```python
from build123d import *

# Parameters (mm, degrees)
SKETCH004_W                 = 51
SKETCH004_H                 = 35.4
PAD002_DEPTH                = 23.5
THICKNESS001_T              = 2
POCKET002_DEPTH             = 55.001
POCKET003_DEPTH             = 2
POCKET004_DEPTH             = 2
POCKET005_DEPTH             = 2
SKETCH009_W                 = 6
SKETCH009_H                 = 2.4
PAD003_DEPTH                = 0.5
SKETCH010_R                 = 1.2
POCKET006_DEPTH             = 2
SKETCH011_W                 = 10
SKETCH011_H                 = 3
PAD004_DEPTH                = 23.5
SKETCH011_POLARPATTERN_2_W  = 10
SKETCH011_POLARPATTERN_2_H  = 3
PAD004_POLARPATTERN_2_DEPTH = 23.5
SKETCH022_W                 = 10
SKETCH022_H                 = 0.15
POCKET013_DEPTH             = 7.1
SKETCH013_R                 = 1.1
SKETCH013_W                 = 10
SKETCH013_H                 = 3.02
PAD005_DEPTH                = 5
SKETCH014_W                 = 2.2
SKETCH014_H                 = 17.18
SKETCH014_H_2               = 17.78
PAD006_DEPTH                = 2.4
SKETCH019_R                 = 0.6
POCKET010_DEPTH             = 42.301
FILLET001_R                 = 1.85
FILLET002_R                 = 1.5


with BuildPart() as part:
    # Sketch004 → Pad002 (new body)
    with BuildSketch(Plane.XY):
        Rectangle(SKETCH004_W, SKETCH004_H)
    extrude(amount=PAD002_DEPTH)

    # Thickness001
    thickness001_openings = [part.faces().sort_by_distance(p)[0] for p in [
        (0, 0, 0),
    ]]
    offset(amount=THICKNESS001_T, openings=thickness001_openings)

    # Sketch005 (on DatumPlane) → Pocket002 (cut, through all)
    with BuildSketch(Plane.YZ.offset(27.5)):
        with BuildLine():
            Line((17.046003, 7.1), (13.527395, 1.798614))
            ThreePointArc((10.361297, 0.1), (12.157784, 0.551473), (13.527395, 1.798614))
            Line((10.361297, 0.1), (-10.361297, 0.1))
            ThreePointArc((-13.527395, 1.798614), (-12.157784, 0.551473), (-10.361297, 0.1))
            Line((-13.527395, 1.798614), (-17.046003, 7.1))
            Line((-17.046003, 7.1), (-40, 7.1))
            Line((-40, 7.1), (-40, -32.9))
            Line((-40, -32.9), (40, -32.9))
            Line((40, -32.9), (40, 7.1))
            Line((40, 7.1), (17.046003, 7.1))
        make_face()
    extrude(amount=-POCKET002_DEPTH, mode=Mode.SUBTRACT)

    # Sketch006 (on DatumPlane) → Pocket003 (cut)
    with BuildSketch(Plane.YZ.offset(-27.5)):
        with BuildLine():
            ThreePointArc((6.4, 6.5), (6.107107, 7.207107), (5.4, 7.5))
            Line((-5.4, 7.5), (5.4, 7.5))
            ThreePointArc((-5.4, 7.5), (-6.107107, 7.207107), (-6.4, 6.5))
            Line((-6.4, 3.5), (-6.4, 6.5))
            ThreePointArc((-6.4, 3.5), (-6.107107, 2.792893), (-5.4, 2.5))
            Line((5.4, 2.5), (-5.4, 2.5))
            ThreePointArc((5.4, 2.5), (6.107107, 2.792893), (6.4, 3.5))
            Line((6.4, 6.5), (6.4, 3.5))
        make_face()
    extrude(amount=POCKET003_DEPTH, mode=Mode.SUBTRACT)

    # Sketch007 (on DatumPlane) → Pocket004 (cut)
    with BuildSketch(Plane.YZ.offset(27.5)):
        with BuildLine():
            ThreePointArc((-7, 21), (-7.707107, 20.707107), (-8, 20))
            Line((-8, 10), (-8, 20))
            ThreePointArc((-8, 10), (-7.707107, 9.292893), (-7, 9))
            Line((7, 9), (-7, 9))
            ThreePointArc((7, 9), (7.707107, 9.292893), (8, 10))
            Line((8, 20), (8, 10))
            ThreePointArc((8, 20), (7.707107, 20.707107), (7, 21))
            Line((-7, 21), (7, 21))
        make_face()
    extrude(amount=-POCKET004_DEPTH, mode=Mode.SUBTRACT)

    # Sketch008 (on DatumPlane) → Pocket005 (cut)
    with BuildSketch(Plane.XY.offset(25.5)):
        Polygon((-5.5, 15.8), (-4.5, 15.8), (-4.5, 1.8), (4.5, 1.8), (4.5, 15.8), (5.5, 15.8), (5.5, 0.8), (-5.5, 0.8), align=None)
        Polygon((-5.5, -0.8), (5.5, -0.8), (5.5, -15.8), (4.5, -15.8), (4.5, -1.8), (-4.5, -1.8), (-4.5, -15.8), (-5.5, -15.8), align=None)
    extrude(amount=-POCKET005_DEPTH, mode=Mode.SUBTRACT)

    # Sketch009 (on Face4 of Pocket005) → Pad003 (join)
    with BuildSketch(Plane(origin=(0, 0, 23.5), x_dir=(1, 0, 0), z_dir=(0, 0, -1))):
        with Locations((0, -3)):
            Rectangle(SKETCH009_W, SKETCH009_H)
        with Locations((0, 3)):
            Rectangle(SKETCH009_W, SKETCH009_H)
    extrude(amount=PAD003_DEPTH)

    # Sketch010 (on DatumPlane) → Pocket006 (cut)
    with BuildSketch(Plane.XY.offset(25.5)):
        with Locations((19, 3)):
            Circle(SKETCH010_R)
        with Locations((9, 3)):
            Circle(SKETCH010_R)
        with Locations((-9, 3)):
            Circle(SKETCH010_R)
        with Locations((-19, 3)):
            Circle(SKETCH010_R)
        with Locations((-19, -3)):
            Circle(SKETCH010_R)
        with Locations((-9, -3)):
            Circle(SKETCH010_R)
        with Locations((9, -3)):
            Circle(SKETCH010_R)
        with Locations((19, -3)):
            Circle(SKETCH010_R)
    extrude(amount=-POCKET006_DEPTH, mode=Mode.SUBTRACT)

    # Sketch011 (on DatumPlane) → Pad004 (join)
    with BuildSketch(Plane.XY.offset(23.5)):
        with Locations((19.5, -16.2)):
            Rectangle(SKETCH011_W, SKETCH011_H)
    pad004 = extrude(amount=-PAD004_DEPTH)

    # Sketch011 PolarPattern 2 → Pad004 PolarPattern 2 (add)
    with BuildSketch(Plane(origin=(0, 0, 23.5), x_dir=(-1, 0, 0), z_dir=(0, 0, 1))):
        with Locations((19.5, -16.2)):
            Rectangle(SKETCH011_POLARPATTERN_2_W, SKETCH011_POLARPATTERN_2_H)
    pad004_polarpattern_2 = extrude(amount=-PAD004_POLARPATTERN_2_DEPTH)

    # Mirrored: Pad004, Pad004 PolarPattern 2 across Sketch011 V_Axis
    add(pad004.mirror(Plane(origin=(0, 0, 23.5), x_dir=(0, 0, 1), z_dir=(1, 0, 0))))
    add(pad004_polarpattern_2.mirror(Plane(origin=(0, 0, 23.5), x_dir=(0, 0, 1), z_dir=(1, 0, 0))))

    # Sketch022 (on DatumPlane) → Pocket013 (cut)
    with BuildSketch(Plane(origin=(0, 0, 0), x_dir=(-1, 0, 0), z_dir=(0, 0, -1))):
        with Locations((19.5, -17.625)):
            Rectangle(SKETCH022_W, SKETCH022_H)
        with Locations((-19.5, -17.625)):
            Rectangle(SKETCH022_W, SKETCH022_H)
        with Locations((19.5, 17.625)):
            Rectangle(SKETCH022_W, SKETCH022_H)
        with Locations((-19.5, 17.625)):
            Rectangle(SKETCH022_W, SKETCH022_H)
    extrude(amount=-POCKET013_DEPTH, mode=Mode.SUBTRACT)

    # Sketch013 (on DatumPlane) → Pad005 (join)
    with BuildSketch(Plane.XY.offset(23.5)):
        with Locations((-22.86, -8.59)):
            Circle(SKETCH013_R)
        with Locations((22.86, -8.89)):
            Circle(SKETCH013_R)
        with Locations((22.86, 8.89)):
            Circle(SKETCH013_R)
        with Locations((-22.86, 8.59)):
            Circle(SKETCH013_R)
        with Locations((-19.5, 13.19)):
            Rectangle(SKETCH013_W, SKETCH013_H)
        with Locations((-19.5, -13.19)):
            Rectangle(SKETCH013_W, SKETCH013_H)
        with Locations((19.5, -13.19)):
            Rectangle(SKETCH013_W, SKETCH013_H)
        with Locations((19.5, 13.19)):
            Rectangle(SKETCH013_W, SKETCH013_H)
    extrude(amount=-PAD005_DEPTH)

    # Sketch014 (on DatumPlane) → Pad006 (join)
    with BuildSketch(Plane.XY.offset(23.5)):
        with Locations((-22.86, 0)):
            Rectangle(SKETCH014_W, SKETCH014_H)
        with Locations((22.86, 0)):
            Rectangle(SKETCH014_W, SKETCH014_H_2)
    extrude(amount=-PAD006_DEPTH)

    # Sketch019 (on DatumPlane) → Pocket010 (cut, through all)
    with BuildSketch(Plane.XZ.offset(22.6)):
        with Locations((-19.5, 3.5)):
            Circle(SKETCH019_R)
        with Locations((19.5, 3.5)):
            Circle(SKETCH019_R)
    extrude(amount=-POCKET010_DEPTH, mode=Mode.SUBTRACT)

    # Fillet001
    fillet001_edges = [part.edges().sort_by_distance(p)[0] for p in [
        (0, -17.7, 23.5),
        (0, 17.7, 23.5),
    ]]
    fillet(fillet001_edges, radius=FILLET001_R)

    # Fillet002
    fillet002_edges = [part.edges().sort_by_distance(p)[0] for p in [
        (-25.5, 0, 23.5),
        (25.5, 0, 23.5),
    ]]
    fillet(fillet002_edges, radius=FILLET002_R)


with BuildPart() as part_1:
    # Body002 placement: moved
    add(part.part.moved(Location((0, 0, 7))))


solid = part_1.part
```
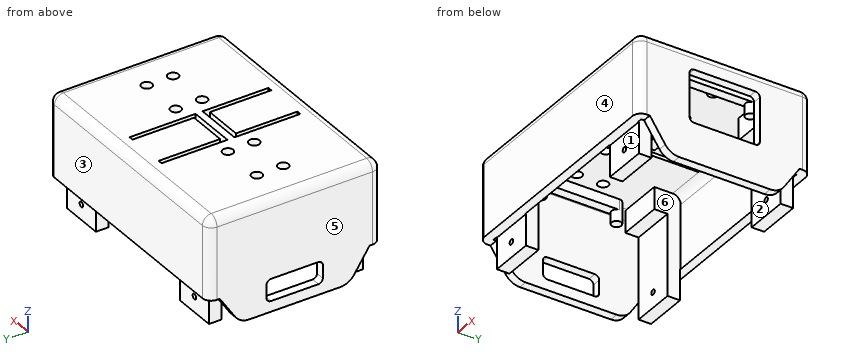
For this review, take the finished solid that the model builds, in its own axes (mm). Face numbers are marked on the shaded views. A direction names the side the tool comes from. Coordinates: 2 decimals unless noted, no trailing zeros. Order: outer loops, then holes, each group sorted by start corner. A loop starts at its lowest first (then second) coordinate and runs counter-clockwise, first axis right, second up. Notation, with made-up numbers: (48, 47.5) - (103, 47.5) arc R8 cw to (103, 61.5) - close; hole circle Ø5 at (11, 39.25). An arc over 180 degrees is marked (long way). Answer as a JSON object with one key per item and string values. Group by question number.
1. For the marked faces 1, 2 and 3, list the 3-axis set-ups (+Z, -Z, +X, -X, +Y, -Y) from which the entire face can be reached by the end or side of a thin tool; tool diameter is ignored.
2. The part is to be moulded in two halves that separate along X. For the marked faces 4, 5 and 6, say which applies: pulls with the +X half, pulls with the -X half, needs draft (parallel to the pull), parting line crosses it, or undercut.
3. We need section D-D on x = 22.86. State the section outline as (y, z) points, then the cut area to 3 significant figures.
4. We need section A-A on x = 9. State the section outline as (y, z) points, then the cut area to 3 significant figures.
5. We need section B-B on y = 0. Give the number of separate pieces and of enclosed holes in the cut face, then the cut area to 3 significant figures.
6. For probe 1 along X at (y, z) = (-11, 27); probe 2 along Y at (x, z) = (-9, 31.2); probe 3 along Y at (x, z) = (23.5, 9), list the stretches that pass through material, from the lowest coordinate up.
7. Clearance check with flat-ended pins moving along their axes: P1, Ø1.5, axis at x = 18.5, y = -12.5, coming from the -Z side; P2, Ø2, axis at x = -17.5, z = 10, coming from the +Y side; P3, Ø1.6, axis at x = -27, z = 11.5, coming from the +Y side. State where each tip first meets the part, or that it passes through.
Final values:
{
 "1": {"face 1": "-Z, +X, -X, -Y", "face 2": "-Z", "face 3": "+Z, -Z, +X, -X, +Y"},
 "2": {"face 4": "needs draft", "face 5": "pulls with the -X half", "face 6": "undercut"},
 "3": {"outline": "(-19.7, 14.1) - (-17.55, 14.1) - (-17.55, 7) - (-14.7, 7) - (-14.7, 25.5) - (-11.68, 25.5) - (-11.68, 30.5) - (-9.99, 30.5) - (-9.99, 25.5) - (-7.79, 25.5) - (-7.79, 28.1) - (7.79, 28.1) - (7.79, 25.5) - (9.99, 25.5) - (9.99, 30.5) - (11.68, 30.5) - (11.68, 25.5) - (14.7, 25.5) - (14.7, 7) - (17.55, 7) - (17.55, 14.1) - (19.7, 14.1) - (19.7, 30.5) arc R2 ccw to (17.7, 32.5) - (-17.7, 32.5) arc R2 ccw to (-19.7, 30.5) - close", "area": "371 mm²"},
 "4": {"outline": "(-19.7, 14.1) - (-17.7, 14.1) - (-17.7, 28.65) arc R1.85 cw to (-15.85, 30.5) - (-4.2, 30.5) - (-4.2, 32.5) - (-17.7, 32.5) arc R2 ccw to (-19.7, 30.5) - close; (-1.8, 30.5) - (1.8, 30.5) - (1.8, 32.5) - (-1.8, 32.5) - close; (4.2, 30.5) - (15.85, 30.5) arc R1.85 cw to (17.7, 28.65) - (17.7, 14.1) - (19.7, 14.1) - (19.7, 30.5) arc R2 ccw to (17.7, 32.5) - (4.2, 32.5) - close", "area": "135 mm²"},
 "5": {"separate pieces": "3", "enclosed holes": "0", "area": "179 mm²"},
 "6": {"probe 1": "-27.5 to -25.5, 25.5 to 27.5", "probe 2": "-19.57 to -4.2, -1.8 to 1.8, 4.2 to 19.57", "probe 3": "-17.55 to -14.7, 14.7 to 17.55"},
 "7": {"P1": "z = 25.5", "P2": "y = 17.55", "P3": "y = 15.85"}
}
